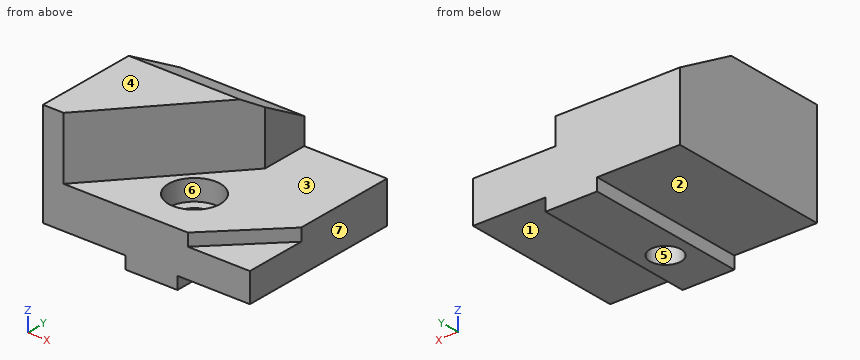
```python
from build123d import *

# Parameters (mm, degrees)
SKETCH_W        = 100
SKETCH_H        = 80
PAD_DEPTH       = 56
SKETCH001_W     = 40
SKETCH001_H     = 99.175636
SKETCH001_W_2   = 35
SKETCH001_H_2   = 102.941795
POCKET_DEPTH    = 6
POCKET001_DEPTH = 30
SKETCH003_R     = 7.5
POCKET002_DEPTH = 26.001
SKETCH004_R     = 12.5
POCKET003_DEPTH = 10
POCKET004_DEPTH = 6
POCKET005_DEPTH = 100.001
SKETCH007_W     = 20
SKETCH007_H     = 31.79351
POCKET006_DEPTH = 80.001


with BuildPart() as part:
    # Sketch → Pad (new body)
    with BuildSketch(Plane.XY):
        Rectangle(SKETCH_W, SKETCH_H)
    extrude(amount=PAD_DEPTH)

    # Sketch001 → Pocket (cut)
    with BuildSketch(Plane(origin=(0, 0, 0), x_dir=(1, 0, 0), z_dir=(0, 0, -1))):
        with Locations((-30, -1.79467)):
            Rectangle(SKETCH001_W, SKETCH001_H)
        with Locations((32.5, -0.915902)):
            Rectangle(SKETCH001_W_2, SKETCH001_H_2)
    extrude(amount=-POCKET_DEPTH, mode=Mode.SUBTRACT)

    # Sketch002 → Pocket001 (cut)
    with BuildSketch(Plane.XY.offset(56)):
        Polygon((-40, -40), (30, 40), (50, 40), (50, -40), align=None)
    extrude(amount=-POCKET001_DEPTH, mode=Mode.SUBTRACT)

    # Sketch003 → Pocket002 (cut, through all)
    with BuildSketch(Plane.XY.offset(26)):
        with Locations((2.5, -15)):
            Circle(SKETCH003_R)
    extrude(amount=-POCKET002_DEPTH, mode=Mode.SUBTRACT)

    # Sketch004 → Pocket003 (cut)
    with BuildSketch(Plane.XY.offset(26)):
        with Locations((2.5, -15)):
            Circle(SKETCH004_R)
    extrude(amount=-POCKET003_DEPTH, mode=Mode.SUBTRACT)

    # Sketch005 → Pocket004 (cut)
    with BuildSketch(Plane.XY.offset(26)):
        Polygon((20, -40), (50, -10), (50, -40), align=None)
    extrude(amount=-POCKET004_DEPTH, mode=Mode.SUBTRACT)

    # Sketch006 → Pocket005 (cut, through all)
    with BuildSketch(Plane(origin=(-50, 0, 0), x_dir=(0, -1, 0), z_dir=(-1, 0, 0))):
        Polygon((-40, 38.679492), (-40, 56), (-10, 56), align=None)
    extrude(amount=-POCKET005_DEPTH, mode=Mode.SUBTRACT)

    # Sketch007 → Pocket006 (cut, through all)
    with BuildSketch(Plane(origin=(0, 40, 0), x_dir=(-1, 0, 0), z_dir=(0, 1, 0))):
        with Locations((-20, 41.896755)):
            Rectangle(SKETCH007_W, SKETCH007_H)
    extrude(amount=-POCKET006_DEPTH, mode=Mode.SUBTRACT)


solid = part.part
```
Work out the finished part from the listing and answer in its coordinate system (mm). Face numbers are marked on the shaded views. A direction names the side the tool comes from. Round coordinates to 2 decimals unless told otherwise and drop trailing zeros. Write each loop counter-clockwise with the first axis right and the second up, starting at its lowest first coordinate (ties: lowest second). Pieces come first, ordered by that corner, then holes.
1) Flat-ended cylindrical pins translate along their axes: P1, Ø5, axis at y = 1.5, z = 43, coming from the +X side; P2, Ø8, axis at x = 14, y = 8.5, coming from the +Z side; P3, Ø6.5, axis at y = -10, z = 2, coming from the -X side. Find the tip coordinate at first contact, or state that the pin passes through.
2) A cutting plane is placed at C-C on x = 6. Determine the outline of the cut face in (y, z), and give its area (3 significant figures).
3) Consider probe 1 along Y at (x, z) = (2.5, 23); probe 2 along Z at (x, y) = (20, 30); probe 3 along Z at (x, y) = (13, 23). Determine where each line is inside the solid, lowest interval first.
4) Which of the six approach directions +Z, -Z, +X, -X, +Y, -Y give full straight-line access (tool end or side, diameter ignored) to the marked faces 1, 2 and 3?
5) A cutting plane is placed at A-A on y = -15. Determine the outline of the cut face in (x, z) (3 decimals), and give its area (3 significant figures).
6) A cutting plane is placed at B-B on z = 22.5. Determine the outline of the cut face in (x, y), and give its area (3 significant figures).
7) A cutting plane is placed at D-D on y = 0. Determine the outline of the cut face in (x, z), and give its area (3 significant figures).
8) Determine the mould class of the marked faces 4, 5, 6 and 7 for opening direction X: pulls with the +X half, pulls with the -X half, needs draft (parallel to the pull), parting line crosses it, or undercut.
Entries:
1. P1: stops at x = -1.5
1. P2: stops at z = 26
1. P3: stops at x = -10
2. outline: (-40, 0) - (-21.63, 0) - (-21.63, 16) - (-27, 16) - (-27, 26) - (-40, 26) - close; (-8.37, 0) - (40, 0) - (40, 38.68) - (12.57, 54.52) - (12.57, 26) - (-3, 26) - (-3, 16) - (-8.37, 16) - close
2. area: 2,190 mm2
3. probe 1: y = -40 to -27.5, -2.5 to 40
3. probe 2: z = 6 to 26
3. probe 3: z = 0 to 26
4. face 1: -Z, +X, +Y, -Y
4. face 2: -Z, -X, +Y, -Y
4. face 3: +Z, +X, -Y
5. outline: (-50, 6) - (-10, 6) - (-10, 0) - (-5, 0) - (-5, 16) - (-10, 16) - (-10, 26) - (-18.125, 26) - (-18.125, 56) - (-50, 56) - close; (10, 0) - (15, 0) - (15, 6) - (50, 6) - (50, 20) - (45, 20) - (45, 26) - (15, 26) - (15, 16) - (10, 16) - close
5. area: 2,590 mm2
6. outline: (-50, -40) - (20, -40) - (50, -10) - (50, 40) - (-50, 40) - close; hole circle Ø25 at (2.5, -15)
6. area: 7,060 mm2
7. outline: (-50, 6) - (-10, 6) - (-10, 0) - (15, 0) - (15, 6) - (50, 6) - (50, 26) - (-5, 26) - (-5, 56) - (-50, 56) - close
7. area: 3,500 mm2
8. face 4: needs draft
8. face 5: undercut
8. face 6: undercut
8. face 7: pulls with the +X half
